```python
from build123d import *

# Parameters (mm, degrees)
SKETCH1_W                  = 250
SKETCH1_H                  = 98
BOSS_EXTRUDE1_DEPTH        = 2
FILLET1_R                  = 6
SKETCH2_W                  = 6.2
SKETCH2_H                  = 22
CUT_EXTRUDE1_DEPTH         = 12
FILLET2_R                  = 2
F_3_5_3_5_DIAMETER_HOLE1_D = 3.5
SKETCH6_R                  = 1.75
SKETCH6_R_2                = 3.855
SKETCH6_R_3                = 12.5
SKETCH6_R_4                = 3
SKETCH6_W                  = 72.8
SKETCH6_H                  = 22.8
SKETCH6_W_2                = 12.9
SKETCH6_H_2                = 19.2
CUT_EXTRUDE2_DEPTH         = 12
FILLET3_R                  = 2


with BuildPart() as part:
    # Sketch1 → Boss-Extrude1 (new body)
    with BuildSketch(Plane.XY):
        Rectangle(SKETCH1_W, SKETCH1_H)
    extrude(amount=BOSS_EXTRUDE1_DEPTH)

    # Fillet1
    fillet1_edges = [part.edges().sort_by_distance(p)[0] for p in [
        (-125, -49, 1),
        (125, -49, 1),
        (125, 49, 1),
        (-125, 49, 1),
    ]]
    fillet(fillet1_edges, radius=FILLET1_R)

    # Sketch2 → Cut-Extrude1 (cut)
    with BuildSketch(Plane.XY.offset(2)):
        with Locations((-125, 0)):
            Rectangle(SKETCH2_W, SKETCH2_H)
        with Locations((125, 0)):
            Rectangle(SKETCH2_W, SKETCH2_H)
    extrude(amount=-CUT_EXTRUDE1_DEPTH, mode=Mode.SUBTRACT)

    # Fillet2
    fillet2_edges = [part.edges().sort_by_distance(p)[0] for p in [
        (-121.9, 11, 1),
        (-121.9, -11, 1),
        (121.9, 11, 1),
        (121.9, -11, 1),
    ]]
    fillet(fillet2_edges, radius=FILLET2_R)

    # Ø3.5 (3.5) Diameter Hole1 (through all)
    with Locations(Plane.XY.offset(2)):
        with Locations((-120.52, 33.75), (-120.52, -33.75), (120.52, -33.75), (120.52, 33.75)):
            Hole(F_3_5_3_5_DIAMETER_HOLE1_D / 2)

    # Sketch6 → Cut-Extrude2 (cut)
    with BuildSketch(Plane.XY.offset(2)):
        with Locations((-77, 17)):
            Circle(SKETCH6_R)
        with Locations((-77, -17)):
            Circle(SKETCH6_R)
        with Locations((97, 17)):
            Circle(SKETCH6_R)
        with Locations((97, -17)):
            Circle(SKETCH6_R)
        with Locations((-72, 0)):
            Circle(SKETCH6_R)
        with Locations((-63.5, 0)):
            Circle(SKETCH6_R_2)
        with Locations((55, 0)):
            Circle(SKETCH6_R_3)
        with Locations((80, 0)):
            Circle(SKETCH6_R_4)
        with Locations((-13.6, 0)):
            Rectangle(SKETCH6_W, SKETCH6_H)
        with Locations((-100, 0)):
            Rectangle(SKETCH6_W_2, SKETCH6_H_2)
    extrude(amount=-CUT_EXTRUDE2_DEPTH, mode=Mode.SUBTRACT)

    # Fillet3
    fillet3_edges = [part.edges().sort_by_distance(p)[0] for p in [
        (22.8, 11.4, 1),
        (22.8, -11.4, 1),
        (-50, -11.4, 1),
        (-50, 11.4, 1),
        (-93.55, 9.6, 1),
        (-93.55, -9.6, 1),
        (-106.45, -9.6, 1),
        (-106.45, 9.6, 1),
    ]]
    fillet(fillet3_edges, radius=FILLET3_R)


solid = part.part
```
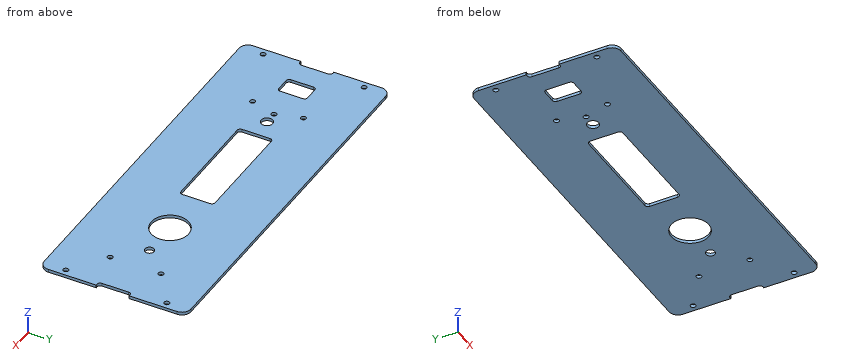
The listing builds one solid part. Answer for the finished solid, in the listing's coordinates (mm). Round coordinates to 2 decimals unless told otherwise and drop trailing zeros. Write each loop counter-clockwise with the first axis right and the second up, starting at its lowest first coordinate (ties: lowest second). Pieces come first, ordered by that corner, then holes. Notation, with made-up numbers: (-38, -22) -> (2, -22) arc R26 ccw to (2, 11) -> close; hole circle Ø6 at (17, 75.5). An arc over 180 degrees is marked (long way). Use CSV: the item, a comma, the result in double quotes. Start each with the question number.
(1) Section A-A on x = -7 is taken. Give the vertices of the cut face in (y, z), then the cut area to 3 significant figures.
(2) Consider L1, parallel to Y at x = -77, z = 1.65; L2, parallel to Y at x = 80, z = 0.95; L3, parallel to Y at x = -28, z = 0.4. Determine where each line is inside the solid, lowest interval first. Write a range as from..to.
(3) Each of these flat-tipped pins is pushed along its axis until it touches: pin 1 (5.5 mm diameter, centred on x = 120.52, y = 33.75, fed in from +Z); pin 2 (0.5 mm diameter, centred on x = 124.5, z = 1.5, fed in from +Y); pin 3 (0.9 mm diameter, centred on x = -124.5, z = 0.5, fed in from -Y); pin 4 (1.2 mm diameter, centred on x = -124, z = 1, fed in from +Y). Where does it stop, or does it pass through?
(4) Section C-C on z = 1.3 is taken. Count the separate pieces of the cut face and the enclosed holes in it, then the cut area to 3 significant figures.
(5) Section B-B on x = -63.5 is taken. Give the vertices of the cut face in (y, z) (3 decimals), then the cut area to 3 significant figures.
A:
1,outline,"(-49, 0) -> (-11.4, 0) -> (-11.4, 2) -> (-49, 2) -> close; (11.4, 0) -> (49, 0) -> (49, 2) -> (11.4, 2) -> close"
1,area,"150 mm²"
2,L1,"y = -49..-18.75, -15.25..15.25, 18.75..49"
2,L2,"y = -49..-3, 3..49"
2,L3,"y = -49..-11.4, 11.4..49"
3,pin 1,"stops at z = 2"
3,pin 2,"stops at y = 45.9"
3,pin 3,"stops at y = -46.24"
3,pin 4,"stops at y = 47.08"
4,separate pieces,"1"
4,enclosed holes,"14"
4,area,"21,800 mm²"
5,outline,"(-49, 0) -> (-3.855, 0) -> (-3.855, 2) -> (-49, 2) -> close; (3.855, 0) -> (49, 0) -> (49, 2) -> (3.855, 2) -> close"
5,area,"181 mm²"
